Input: dimensioned drawing with shaded views. Units: mm. Origin: part minimum x, y, z. Coordinates: 2 decimals unless noted, no trailing zeros. Order: outer loops, then holes, each group sorted by start corner. A loop starts at its lowest first (then second) coordinate and runs counter-clockwise, first axis right, second up. Notation, with made-up numbers: (24, 65.25) - (30, 65.25) arc R32 cw to (30, 98.25) - close; hole circle Ø10 at (66, 68.5). An arc over 180 degrees is marked (long way). One line per question, with ' | ' between items. Start each with the question number.
(1) Section D-D (z = 122.5). Return the cut outline in (x, y) (1 decimal), then the cut area to 3 significant figures.
(2) Line query: line 1 along X through (y, z) = (5, 174) (1 decimal); line 2 along X through (y, z) = (6.5, 142) (1 decimal). Output: solid intervals per line, ascending.
(3) Section B-B (y = 16.5). Return the cut outline in (x, z) (1 decimal), then the cut area to 3 significant figures.
(4) Contact query for flat-ended pins moving along their axis: P1, Ø6, axis at y = 3.5, z = 171, coming from the -X side; P2, Ø10, axis at y = 17.5, z = 155.5, coming from the -X side (1 decimal); P3, Ø4, axis at x = 149.5, y = 3.5, coming from the -Z side (1 decimal). Output: stop coordinate, or through.
(5) Section C-C (x = 49). Return the cut outline in (y, z) (1 decimal), then the cut area to 3 significant figures.
(6) Draft query along Z for the marked faces 1, 2 and 3. Return one class per face: +Z half, -Z half, draft (parallel to the pull), parting line (faces both ways), or undercut.
(7) Section A-A (z = 35). Return the cut outline in (x, y).
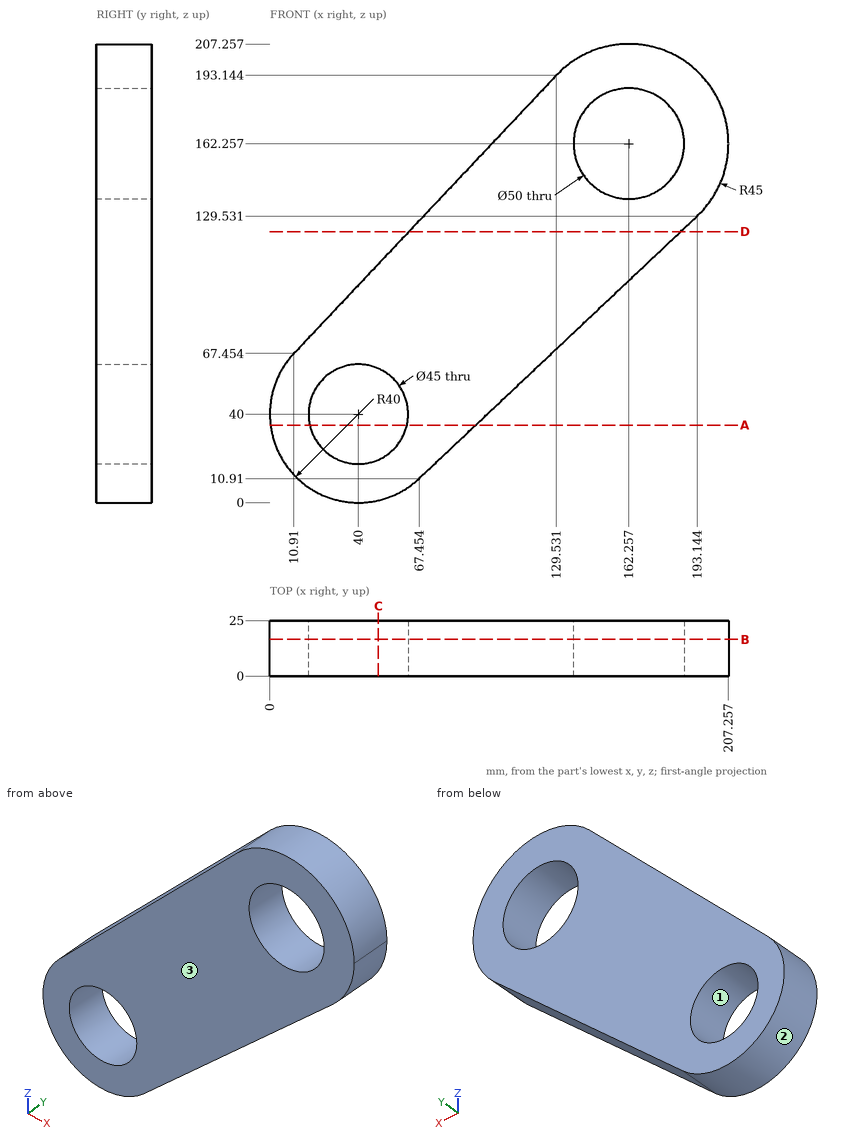
Response values:
1) outline: (62.9, 0) - (185.7, 0) - (185.7, 25) - (62.9, 25) - close | area: 3,070 mm²
2) line 1: x = 111.5 to 140.2, 184.3 to 205.7 | line 2: x = 81.3 to 147.6, 176.9 to 202.4
3) outline: (10.9, 67.5) arc R40 ccw to (67.5, 10.9) - (193.1, 129.5) arc R45 ccw to (207.3, 162.3) arc R45 ccw to (129.5, 193.1) - close; hole circle Ø45 at (40, 40); hole circle Ø50 at (162.3, 162.3) | area: 16,800 mm²
4) P1: stops at x = 105.8 | P2: stops at x = 89.3 | P3: stops at z = 86.5
5) outline: (0, 1) - (25, 1) - (25, 19.4) - (0, 19.4) - close; (0, 60.6) - (25, 60.6) - (25, 107.8) - (0, 107.8) - close | area: 1,640 mm²
6) face 1: undercut | face 2: parting line | face 3: draft
7) outline: (0.31, 0) - (18.06, 0) - (18.06, 25) - (0.31, 25) - close; (61.94, 0) - (92.98, 0) - (92.98, 25) - (61.94, 25) - close
